Part model, mm, in its own coordinate system. Face numbers are marked on the shaded views. A direction names the side the tool comes from. Coordinates: 2 decimals unless noted, no trailing zeros. Loops run counter-clockwise (first coordinate to the right, second up) from the corner with the lowest first, then second, coordinate; pieces in that order, holes last. Notation, with made-up numbers: (14, 24) -> (48, 24) arc R23 ccw to (48, 45) -> close; hole circle Ø9 at (21.25, 22). An arc over 180 degrees is marked (long way). One line per question, with ' | ' between items. Start each with the question number.
1) Cut at C-C (z = 0). List the corners of the cut face in (x, y), plus the area to 3 significant figures.
2) 3-axis set-ups, long thin cutter, end or side, ignore diameter. For the marked faces 1, 2, 3 and 4: which of +Z, -Z, +X, -X, +Y, -Y reach the whole face in a straight line?
3) Two-plate mould, pull along Z, no slides. Class the marked faces 5, 6 and 7: released by +Z, released by -Z, zero draft, split by the parting line, or undercut.
4) Drop flat-ended pins along their axis: pin 1 (7 mm diameter, centred on x = -14, y = 7.65, fed in from -Z); pin 2 (5 mm diameter, centred on y = 8.5, z = -27.5, fed in from +X); pin 3 (6.5 mm diameter, centred on x = -2, y = 8.5, fed in from -Z). Give the stop position or say it passes through.
5) Cut at A-A (z = -26). List the corners of the cut face in (x, y), plus the area to 3 significant figures.
6) Cut at D-D (y = 2.25). Count the separate pieces of the cut face and the enclosed holes in it, plus the area to 3 significant figures.
7) Probe L1, parallel to X at y = 12, z = 19.5; L2, parallel to X at y = 10.5, z = 0; L3, parallel to X at y = 1.25, z = -20. List the from-to ranges inside material, lowest first. Write a range as from..to.
8) Cut at B-B (x = 0). List the corners of the cut face in (y, z), plus the area to 3 significant figures.
from build123d import *

# Parameters (mm, degrees)
SKETCH_1_W               = 45
SKETCH_1_H               = 45
EXTRUDE_1_DEPTH          = 15.3
SKETCH_2_R               = 19.1
CUT_EXTRUDE_1_DEPTH      = 36.307081443
SKETCH_5_W               = 15
SKETCH_5_H               = 15.3
EXTRUDE_2_DEPTH          = 12
SKETCH_6_R               = 3
CUT_EXTRUDE_4_DEPTH      = 35
SKETCH_7_R               = 1.5
CUT_EXTRUDE_5_DEPTH      = 44.938479832
CUT_EXTRUDE_6_DEPTH      = 6
CUT_EXTRUDE_6_DEPTH_BACK = 6
SKETCH_9_R               = 4.25
CUT_EXTRUDE_7_DEPTH      = 12
CHAMFER_2_SIZE           = 1
CHAMFER_3_SIZE           = 1
CHAMFER_4_SIZE           = 1


# Some blends are built 0.0001 mm under size
with BuildPart() as part:
    # 草图1 → 凸台-拉伸1 (new body)
    with BuildSketch(Plane(origin=(0, 0, 0), x_dir=(1, 0, 0), z_dir=(0, 1, 0))):
        Rectangle(SKETCH_1_W, SKETCH_1_H)
    extrude(amount=EXTRUDE_1_DEPTH)

    # 草图2 → 切除-拉伸1 (cut, through all)
    with BuildSketch(Plane(origin=(0, 15.3, 0), x_dir=(1, 0, 0), z_dir=(0, 1, 0))):
        with Locations(Location((0, 0, 0), (0, 0, 270))):
            Circle(SKETCH_2_R)
    extrude(amount=-CUT_EXTRUDE_1_DEPTH, mode=Mode.SUBTRACT)

    # 草图5 → 凸台-拉伸2 (add)
    with BuildSketch(Plane(origin=(0, 0, -22.5), x_dir=(-1, 0, 0), z_dir=(0, 0, -1))):
        with Locations((14, 7.65)):
            Rectangle(SKETCH_5_W, SKETCH_5_H)
        with Locations((-14, 7.65)):
            Rectangle(SKETCH_5_W, SKETCH_5_H)
    extrude(amount=EXTRUDE_2_DEPTH)

    # 草图6 → 切除-拉伸4 (cut)
    with BuildSketch(Plane(origin=(0, 0, -34.5), x_dir=(-1, 0, 0), z_dir=(0, 0, -1))):
        with Locations((-14, 7.65)):
            Circle(SKETCH_6_R)
        with Locations((14, 7.65)):
            Circle(SKETCH_6_R)
    extrude(amount=-CUT_EXTRUDE_4_DEPTH, mode=Mode.SUBTRACT)

    # 草图7 → 切除-拉伸5 (cut, through all)
    with BuildSketch(Plane(origin=(0, 15.3, 0), x_dir=(1, 0, 0), z_dir=(0, 1, 0))):
        with Locations(Location((-19.5, 19.5, 0), (0, 0, 270))):
            Circle(SKETCH_7_R)
        with Locations(Location((19.5, 19.5, 0), (0, 0, 90))):
            Circle(SKETCH_7_R)
        with Locations(Location((19.5, -19.5, 0), (0, 0, 270))):
            Circle(SKETCH_7_R)
        with Locations(Location((-19.5, -19.5, 0), (0, 0, 90))):
            Circle(SKETCH_7_R)
    extrude(amount=-CUT_EXTRUDE_5_DEPTH, mode=Mode.SUBTRACT)

    # 草图8 → 切除-拉伸6 (cut, two sides: drawn at the far end of the back side and taken through both)
    with BuildSketch(Plane(origin=(0, 7.65, 0), x_dir=(-1, 0, 0), z_dir=(0, -1, 0)).offset(-CUT_EXTRUDE_6_DEPTH_BACK)):
        with BuildLine():
            Line((-8.874983497, 19.032463528), (-8.072008799, 17.310478732))
            ThreePointArc((-8.072008799, 17.310478732), (-15.1530488, 11.627343294), (-18.809828083, 3.316680193))
            Line((-18.809828083, 3.316680193), (-20.680962813, 3.646611731))
            ThreePointArc((-20.680962813, 3.646611731), (-16.660420146, 12.783990009), (-8.874983497, 19.032463528))
        make_face()
        with BuildLine():
            Line((20.680962813, 3.646611731), (18.809828083, 3.316680193))
            ThreePointArc((18.809828083, 3.316680193), (15.1530488, 11.627343294), (8.072008799, 17.310478732))
            Line((8.072008799, 17.310478732), (8.874983497, 19.032463528))
            ThreePointArc((8.874983497, 19.032463528), (16.660420146, 12.783990009), (20.680962813, 3.646611731))
        make_face()
    extrude(amount=CUT_EXTRUDE_6_DEPTH + CUT_EXTRUDE_6_DEPTH_BACK, mode=Mode.SUBTRACT)

    # 草图9 → 切除-拉伸7 (cut)
    with BuildSketch(Plane(origin=(0, 0, -34.5), x_dir=(-1, 0, 0), z_dir=(0, 0, -1))):
        with Locations((-14, 7.65)):
            Circle(SKETCH_9_R)
        with Locations((14, 7.65)):
            Circle(SKETCH_9_R)
    extrude(amount=-CUT_EXTRUDE_7_DEPTH, mode=Mode.SUBTRACT)

    # 倒角1
    # the kernel refuses this chamfer: 2 mm, written as the material it takes off along each edge
    with BuildSketch(Plane(origin=(-18.809828083, 1.65, -3.316680193), x_dir=(-0.09666023054018325, 0, 0.9953174367165073), z_dir=(0, 1, 0))) as chamfer_1_piece_1_section:
        with BuildLine():
            Line((1.811638226, -0.054831322), (-0.147910468, -1.899248595))
            Line((-0.147910468, -1.899248595), (0, 0))
            ThreePointArc((0, 0), (0.933514183, -0.049753736), (1.811638226, -0.054831322))
        make_face()
    chamfer_1_piece_1 = extrude(amount=12, mode=Mode.PRIVATE)
    chamfer_1_piece_1 = chamfer_1_piece_1 & Plane(origin=(0, 7.65, 0), x_dir=(-0.42261826174070266, 0, -0.9063077870366485), z_dir=(0, 1, 0)) * Cylinder(21, 32, mode=Mode.PRIVATE)
    add(chamfer_1_piece_1, mode=Mode.SUBTRACT)
    with BuildSketch(Plane(origin=(18.809828083, 13.65, -3.316680193), x_dir=(0.09666023054018283, 0, 0.9953174367165073), z_dir=(0, -1, 0))) as chamfer_1_piece_2_section:
        with BuildLine():
            Line((1.811638226, -0.054831322), (-0.147910468, -1.899248595))
            Line((-0.147910468, -1.899248595), (0, 0))
            ThreePointArc((0, 0), (0.933514183, -0.049753736), (1.811638226, -0.054831322))
        make_face()
    chamfer_1_piece_2 = extrude(amount=12, mode=Mode.PRIVATE)
    chamfer_1_piece_2 = chamfer_1_piece_2 & Plane(origin=(0, 7.65, 0), x_dir=(0.9848077530122075, 0, -0.17364817766693397), z_dir=(0, 1, 0)) * Cylinder(21, 32, mode=Mode.PRIVATE)
    add(chamfer_1_piece_2, mode=Mode.SUBTRACT)

    # 倒角2
    chamfer_2_edges = [part.edges().sort_by_distance(p)[0] for p in [
        (22.5, 7.65, 22.5),
        (-22.5, 7.65, 22.5),
        (-22.5, 7.65, -22.5),
        (22.5, 7.65, -22.5),
    ]]
    chamfer(chamfer_2_edges, length=CHAMFER_2_SIZE - 0.0001)  # a hair under: the kernel refuses the full size

    # 倒角3
    chamfer_3_edges = [part.edges().sort_by_distance(p)[0] for p in [
        (18.25, 7.65, -22.5),
        (-9.75, 7.65, -22.5),
    ]]
    chamfer(chamfer_3_edges, length=CHAMFER_3_SIZE)

    # 倒角4
    chamfer_4_edges = [part.edges().sort_by_distance(p)[0] for p in [
        (6.5, 7.65, -34.5),
        (14, 15.3, -34.5),
        (21.5, 7.65, -34.5),
        (14, 0, -34.5),
        (-21.5, 7.65, -34.5),
        (-14, 15.3, -34.5),
        (-6.5, 7.65, -34.5),
        (-14, 0, -34.5),
    ]]
    chamfer(chamfer_4_edges, length=CHAMFER_4_SIZE)


solid = part.part
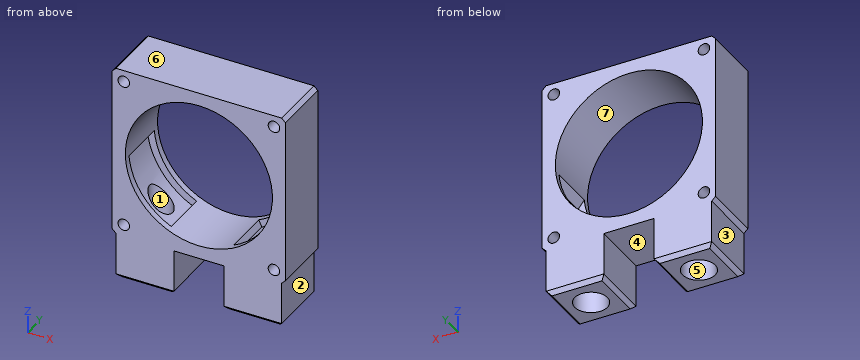
Reported:
1) outline: (-22.5, 0) -> (-19.1, 0) -> (-19.1, 15.3) -> (-22.5, 15.3) -> close; (19.1, 0) -> (22.5, 0) -> (22.5, 15.3) -> (19.1, 15.3) -> close | area: 104 mm²
2) face 1: -Z | face 2: -Z, +X, +Y, -Y | face 3: -Z, -X, +Y, -Y | face 4: -Z, +Y, -Y
3) face 5: zero draft | face 6: released by +Z | face 7: undercut
4) pin 1: stops at z = -22.75 | pin 2: stops at x = 21.5 | pin 3: stops at z = -22.5
5) outline: (-21.5, 0) -> (-6.5, 0) -> (-6.5, 15.3) -> (-21.5, 15.3) -> close; (6.5, 0) -> (21.5, 0) -> (21.5, 15.3) -> (6.5, 15.3) -> close; hole circle Ø8.5 at (-14, 7.65); hole circle Ø8.5 at (14, 7.65) | area: 346 mm²
6) separate pieces: 1 | enclosed holes: 5 | area: 1,130 mm²
7) L1: x = -22.5..-21, -18..18, 21..22.5 | L2: x = -22.5..-19.1, 19.1..22.5 | L3: x = -22.5..-20.91, -18.09..18.09, 20.91..22.5
8) outline: (0, -22.5) -> (15.3, -22.5) -> (15.3, -19.1) -> (0, -19.1) -> close; (0, 19.1) -> (15.3, 19.1) -> (15.3, 22.5) -> (0, 22.5) -> close | area: 104 mm²
